```python
from build123d import *
from build123d.topology import SkipClean

# Parameters (mm, degrees)
BOSS_EXTRUDE1_DEPTH                     = 15
CBORE_FOR_M6_HEX_HEAD_BOLT1_D           = 7
CBORE_FOR_M6_HEX_HEAD_BOLT1_CBORE_D     = 25.6
CBORE_FOR_M6_HEX_HEAD_BOLT1_CBORE_DEPTH = 3
SKETCH30_W                              = 87.8922038
SKETCH30_H                              = 63.386693804
CUT_EXTRUDE8_DEPTH                      = 0.125
SKETCH31_W                              = 82.344977649
SKETCH31_H                              = 39.024548637
CUT_EXTRUDE9_DEPTH                      = 0.125
SKETCH38_R                              = 1.905
CUT_EXTRUDE10_DEPTH                     = 68.319909946
SKETCH39_OUTSIDE_W                      = 91.473
SKETCH39_OUTSIDE_H                      = 49.266
SKETCH39_OUTSIDE_R                      = 12.8
CUT_EXTRUDE11_DEPTH                     = 7.75
SKETCH40_R                              = 13
CUT_EXTRUDE12_DEPTH                     = 6
BOSS_EXTRUDE2_START                     = 4
SKETCH41_R                              = 12.8
BOSS_EXTRUDE2_DEPTH                     = 4
SKETCH42_R                              = 3.5
SKETCH42_R_2                            = 1.905
CUT_EXTRUDE13_DEPTH                     = 67.748958045
SKETCH43_R                              = 14.2
SKETCH43_R_2                            = 12.8
BOSS_EXTRUDE3_DEPTH                     = 8.875
CUT_EXTRUDE14_DEPTH                     = 67.422311011
CUT_EXTRUDE14_DEPTH_BACK                = 4
SKETCH44_R                              = 3.556
SKETCH45_R                              = 1.905
CUT_EXTRUDE15_DEPTH                     = 67.2810184
SKETCH46_R                              = 3.556
CUT_EXTRUDE16_DEPTH                     = 2
SKETCH47_W                              = 10
SKETCH47_H                              = 3.81
CUT_EXTRUDE17_DEPTH                     = 2


with BuildPart() as part:
    # Sketch1 → Boss-Extrude1 (new body)
    with BuildSketch(Plane(origin=(0, 0, 0), x_dir=(-1, 0, 0), z_dir=(0, 0, -1))):
        with BuildLine():
            Line((-54.628463331, -5.212133486), (-0.593380164, -2.525889334))
            ThreePointArc((-0.593380164, -2.525889334), (12.32206912, 15.671805741), (-8.399323253, 23.953643362))
            Line((-8.399323253, 23.953643362), (-43.781031906, 5.260553383))
            ThreePointArc((-43.781031906, 5.260553383), (-45.231601083, 4.760443022), (-46.765522471, 4.723748524))
            Line((-46.765522471, 4.723748524), (-54.189447973, 5.695292216))
            ThreePointArc((-54.189447973, 5.695292216), (-60.376392814, 0.481764046), (-54.628463331, -5.212133486))
        make_face()
    extrude(amount=-BOSS_EXTRUDE1_DEPTH)

    # CBORE for M6 Hex Head Bolt1 (through all)
    with Locations(Plane(origin=(0, 0, 0), x_dir=(-1, 0, 0), z_dir=(0, 0, -1))):
        with Locations((-1.298433566, 11.656596333)):
            CounterBoreHole(CBORE_FOR_M6_HEX_HEAD_BOLT1_D / 2, CBORE_FOR_M6_HEX_HEAD_BOLT1_CBORE_D / 2, CBORE_FOR_M6_HEX_HEAD_BOLT1_CBORE_DEPTH)

    # Sketch30 → Cut-Extrude8 (cut)
    with BuildSketch(Plane.XY.offset(15)):
        with Locations((24.760370948, 9.451685766)):
            Rectangle(SKETCH30_W, SKETCH30_H)
    extrude(amount=-CUT_EXTRUDE8_DEPTH, mode=Mode.SUBTRACT)

    # Sketch31 → Cut-Extrude9 (cut)
    with BuildSketch(Plane(origin=(0, 0, 0), x_dir=(-1, 0, 0), z_dir=(0, 0, -1))):
        with Locations((-23.438477607, 10.614160855)):
            Rectangle(SKETCH31_W, SKETCH31_H)
    extrude(amount=-CUT_EXTRUDE9_DEPTH, mode=Mode.SUBTRACT)

    # Sketch38 → Cut-Extrude10 (cut, through all)
    with BuildSketch(Plane.XY.offset(14.875)):
        with Locations((-5.615950455, 18.571806714)):
            Circle(SKETCH38_R)
        with Locations((8.213643947, 18.570980353)):
            Circle(SKETCH38_R)
        with Locations((8.212817586, 4.741385951)):
            Circle(SKETCH38_R)
        with Locations((-5.616776816, 4.742212313)):
            Circle(SKETCH38_R)
    extrude(amount=-CUT_EXTRUDE10_DEPTH, mode=Mode.SUBTRACT)

    # Sketch39 outside → Cut-Extrude11 (cut)
    with BuildSketch(Plane(origin=(0, 0, 0.125), x_dir=(-1, 0, 0), z_dir=(0, 0, -1))):
        with Locations((-23.7395, 10.319)):
            Rectangle(SKETCH39_OUTSIDE_W, SKETCH39_OUTSIDE_H)
        with Locations(Location((-1.298433566, 11.656596333, 0), (0, 0, 180))):
            Circle(SKETCH39_OUTSIDE_R, mode=Mode.SUBTRACT)
    extrude(amount=-CUT_EXTRUDE11_DEPTH, mode=Mode.SUBTRACT)

    # Sketch40 → Cut-Extrude12 (cut)
    with BuildSketch(Plane.XY.offset(14.875)):
        with Locations((1.298433566, 11.656596333)):
            Circle(SKETCH40_R)
    extrude(amount=-CUT_EXTRUDE12_DEPTH, mode=Mode.SUBTRACT)

    # Sketch41 → Boss-Extrude2 (add)
    with BuildSketch(Plane(origin=(0, 0, 3), x_dir=(-1, 0, 0), z_dir=(0, 0, -1)).offset(BOSS_EXTRUDE2_START)):
        with Locations((-1.298433566, 11.656596333)):
            Circle(SKETCH41_R)
    extrude(amount=-BOSS_EXTRUDE2_DEPTH)

    # Sketch42 → Cut-Extrude13 (cut, through all)
    with BuildSketch(Plane.XY.offset(3)):
        with Locations((1.298433566, 11.656596333)):
            Circle(SKETCH42_R)
        with Locations((8.212817586, 4.741385951)):
            Circle(SKETCH42_R_2)
        with Locations((-5.616776816, 4.742212313)):
            Circle(SKETCH42_R_2)
        with Locations((-5.615950455, 18.571806714)):
            Circle(SKETCH42_R_2)
        with Locations((8.213643947, 18.570980353)):
            Circle(SKETCH42_R_2)
    extrude(amount=-CUT_EXTRUDE13_DEPTH, mode=Mode.SUBTRACT)

    # Sketch43 → Boss-Extrude3 (add, through all)
    with SkipClean():  # the faces are left unmerged after this step: merging them gives an invalid solid
        with BuildSketch(Plane(origin=(0, 0, 7.875), x_dir=(-1, 0, 0), z_dir=(0, 0, -1))):
            with Locations((-1.298433566, 11.656596333)):
                Circle(SKETCH43_R)
            with Locations((-1.298433566, 11.656596333)):
                Circle(SKETCH43_R_2, mode=Mode.SUBTRACT)
        extrude(amount=BOSS_EXTRUDE3_DEPTH)

    # Sketch44 → Cut-Extrude14 (cut, two sides: drawn at the far end of the back side and taken through both)
    with SkipClean():  # the faces are left unmerged after this step: merging them gives an invalid solid
        with BuildSketch(Plane.XY.offset(8.875).offset(-CUT_EXTRUDE14_DEPTH_BACK)):
            with Locations((8.213643947, 18.570980353)):
                Circle(SKETCH44_R)
            with Locations((-5.615950455, 18.571806714)):
                Circle(SKETCH44_R)
            with Locations((-5.616776816, 4.742212313)):
                Circle(SKETCH44_R)
            with Locations((8.212817586, 4.741385951)):
                Circle(SKETCH44_R)
        extrude(amount=CUT_EXTRUDE14_DEPTH + CUT_EXTRUDE14_DEPTH_BACK, mode=Mode.SUBTRACT)

    # Sketch45 → Cut-Extrude15 (cut, through all)
    with SkipClean():  # the faces are left unmerged after this step: merging them gives an invalid solid
        with BuildSketch(Plane(origin=(0, 0, 7.875), x_dir=(-1, 0, 0), z_dir=(0, 0, -1))):
            with Locations((-54.900567232, 0.261366347)):
                Circle(SKETCH45_R)
            with Locations((-44.900567232, 0.261366347)):
                Circle(SKETCH45_R)
        extrude(amount=-CUT_EXTRUDE15_DEPTH, mode=Mode.SUBTRACT)

    # Sketch46 → Cut-Extrude16 (cut)
    with SkipClean():  # the faces are left unmerged after this step: merging them gives an invalid solid
        with BuildSketch(Plane(origin=(0, 0, 7.875), x_dir=(-1, 0, 0), z_dir=(0, 0, -1))):
            with Locations((-54.900567232, 0.261366347)):
                Circle(SKETCH46_R)
            with Locations((-44.900567232, 0.261366347)):
                Circle(SKETCH46_R)
        extrude(amount=-CUT_EXTRUDE16_DEPTH, mode=Mode.SUBTRACT)

    # Sketch47 → Cut-Extrude17 (cut)
    with SkipClean():  # the faces are left unmerged after this step: merging them gives an invalid solid
        with BuildSketch(Plane(origin=(0, 0, 7.875), x_dir=(-1, 0, 0), z_dir=(0, 0, -1))):
            with Locations((-49.900567232, 0.261366347)):
                Rectangle(SKETCH47_W, SKETCH47_H)
        extrude(amount=-CUT_EXTRUDE17_DEPTH, mode=Mode.SUBTRACT)


solid = part.part
```
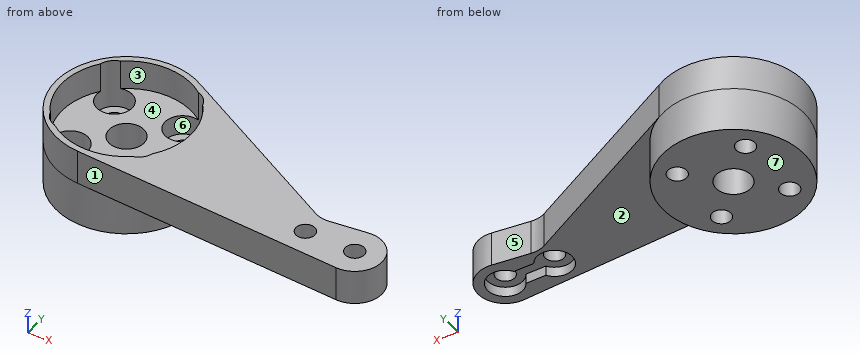
Check sheet for the modelled part. Datum: model origin and axes. Units: mm. Face numbers are marked on the shaded views. A direction names the side the tool comes from. Coordinates: 2 decimals unless noted, no trailing zeros. Write each loop counter-clockwise with the first axis right and the second up, starting at its lowest first coordinate (ties: lowest second). Pieces come first, ordered by that corner, then holes. Notation, with made-up numbers: (15.5, 71) - (22.5, 71) arc R13 cw to (22.5, 89) - close; hole circle Ø9 at (68, 39). An arc over 180 degrees is marked (long way). One line per question, with ' | ' between items.
Item 1: Sectioned sample at A-A on y = -0.5. Record the boundary of the cut face in (x, z) (3 decimals).
Determined:
outline: (-6.04, -1) - (8.637, -1) - (8.637, 7.875) - (41.427, 7.875) - (41.427, 9.875) - (43.154, 9.875) - (43.154, 14.875) - (5.905, 14.875) - (5.905, 8.875) - (-3.308, 8.875) - (-3.308, 14.875) - (-6.04, 14.875) - close; (46.647, 9.875) - (53.154, 9.875) - (53.154, 14.875) - (46.647, 14.875) - close; (56.647, 9.875) - (58.374, 9.875) - (58.374, 7.875) - (60.328, 7.875) - (60.328, 14.875) - (56.647, 14.875) - close
Item 2: Thickness scan on line 1 (Y direction, x = 5.5, z = 8.75); line 2 (X direction, y = 19.5, z = 6.25); line 3 (X direction, y = 20, z = 2.25). Record the ranges inside material, lowest first. Write a range as [from, to].
Determined:
line 1: y = [-2.77, 2.44], [7.04, 16.27], [20.87, 25.22] | line 2: x = [-10.54, -9.05], [-2.18, 4.78], [11.65, 13.14] | line 3: x = [-10.19, -6.88], [-4.36, 6.95], [9.47, 12.79]
Item 3: Sectioned sample at C-C on y = 10. Record the boundary of the cut face in (x, z) (3 decimals), plus the area to 3 significant figures.
Determined:
outline: (-12.805, -1) - (-1.785, -1) - (-1.785, 8.875) - (-11.596, 8.875) - (-11.596, 14.875) - (-12.805, 14.875) - close; (4.382, -1) - (15.401, -1) - (15.401, 7.875) - (34.81, 7.875) - (34.81, 14.875) - (14.192, 14.875) - (14.192, 8.875) - (4.382, 8.875) - close | area: 368 mm2
Item 4: Mould release check, pull along X, two halves, no side actions. Record for the marked faces 1, 2, 3 and 4: pulls with the +X half, pulls with the -X half, needs draft (parallel to the pull), parting line crosses it, or undercut.
Determined:
face 1: pulls with the -X half | face 2: needs draft | face 3: undercut | face 4: undercut
Item 5: Sectioned sample at B-B on z = 3. Record the boundary of the cut face in (x, y) (3 decimals), plus the area to 3 significant figures.
Determined:
outline: circle Ø28.4 at (1.298, 11.657); hole circle Ø3.81 at (-5.617, 4.742); hole circle Ø3.81 at (-5.616, 18.572); hole circle Ø7 at (1.298, 11.657); hole circle Ø3.81 at (8.213, 4.741); hole circle Ø3.81 at (8.214, 18.571) | area: 549 mm2
Item 6: Gauge pin test, flat ends, axial feed: P1, Ø4, axis at x = 15, z = 4, coming from the +Y side; P2, Ø1.6, axis at x = 50.5, z = 9, coming from the +Y side; P3, Ø10, axis at x = -5.5, y = 9, coming from the +Z side (3 decimals). Record the tip position at first contact, or that the pin passes through.
Determined:
P1: stops at y = 19.7 | P2: stops at y = 5.32 | P3: stops at z = 8.875
Item 7: Access from +Z, -Z, +X, -X, +Y, -Y to the whole of each face (thin tool, end or side, straight path). Record for the marked faces 5, 6 and 7.
Determined:
face 5: +Z, -Z, +Y | face 6: +Z | face 7: -Z, +X, -X, +Y, -Y
Item 8: Sectioned sample at D-D on x = 49. Record the boundary of the cut face in (y, z) (3 decimals).
Determined:
outline: (-4.932, 7.875) - (-1.644, 7.875) - (-1.644, 9.875) - (2.166, 9.875) - (2.166, 7.875) - (5.016, 7.875) - (5.016, 14.875) - (-4.932, 14.875) - close
